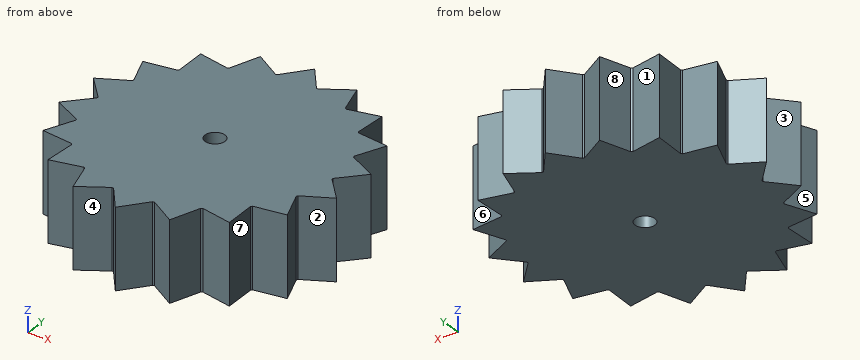
from build123d import *

# Parameters (mm, degrees)
F0_R     = 3.175
F1_DEPTH = 25.4


with BuildPart() as f1:
    # F0 (on Top) → F1 (new body)
    with BuildSketch(Plane.XY):
        with BuildLine():
            Line((0, 45.72), (-6.327913, 37.570833))
            ThreePointArc((-6.327913, 37.570833), (-6.615996, 37.521175), (-6.903689, 37.469309))
            Line((-6.903689, 37.469309), (-15.637161, 42.962747))
            Line((-15.637161, 42.962747), (-18.796275, 33.140761))
            ThreePointArc((-18.796275, 33.140761), (-19.05, 32.995568), (-19.302604, 32.848432))
            Line((-19.302604, 32.848432), (-29.38825, 35.023552))
            Line((-29.38825, 35.023552), (-28.997529, 24.713424))
            ThreePointArc((-28.997529, 24.713424), (-29.186293, 24.490208), (-29.37334, 24.26555))
            Line((-29.37334, 24.26555), (-39.594681, 22.86))
            Line((-39.594681, 22.86), (-35.701253, 13.305283))
            ThreePointArc((-35.701253, 13.305283), (-35.802289, 13.030967), (-35.901217, 12.755885))
            Line((-35.901217, 12.755885), (-45.02541, 7.939195))
            Line((-45.02541, 7.939195), (-38.098879, 0.292329))
            ThreePointArc((-38.098879, 0.292329), (-38.1, 0), (-38.098879, -0.292329))
            Line((-38.098879, -0.292329), (-45.02541, -7.939195))
            Line((-45.02541, -7.939195), (-35.901217, -12.755885))
            ThreePointArc((-35.901217, -12.755885), (-35.802289, -13.030967), (-35.701253, -13.305283))
            Line((-35.701253, -13.305283), (-39.594681, -22.86))
            Line((-39.594681, -22.86), (-29.37334, -24.26555))
            ThreePointArc((-29.37334, -24.26555), (-29.186293, -24.490208), (-28.997529, -24.713424))
            Line((-28.997529, -24.713424), (-29.38825, -35.023552))
            Line((-29.38825, -35.023552), (-19.302604, -32.848432))
            ThreePointArc((-19.302604, -32.848432), (-19.05, -32.995568), (-18.796275, -33.140761))
            Line((-18.796275, -33.140761), (-15.637161, -42.962747))
            Line((-15.637161, -42.962747), (-6.903689, -37.469309))
            ThreePointArc((-6.903689, -37.469309), (-6.615996, -37.521175), (-6.327913, -37.570833))
            Line((-6.327913, -37.570833), (0, -45.72))
            Line((0, -45.72), (6.327913, -37.570833))
            ThreePointArc((6.327913, -37.570833), (6.615996, -37.521175), (6.903689, -37.469309))
            Line((6.903689, -37.469309), (15.637161, -42.962747))
            Line((15.637161, -42.962747), (18.796275, -33.140761))
            ThreePointArc((18.796275, -33.140761), (19.05, -32.995568), (19.302604, -32.848432))
            Line((19.302604, -32.848432), (29.38825, -35.023552))
            Line((29.38825, -35.023552), (28.997529, -24.713424))
            ThreePointArc((28.997529, -24.713424), (29.186293, -24.490208), (29.37334, -24.26555))
            Line((29.37334, -24.26555), (39.594681, -22.86))
            Line((39.594681, -22.86), (35.701253, -13.305283))
            ThreePointArc((35.701253, -13.305283), (35.802289, -13.030967), (35.901217, -12.755885))
            Line((35.901217, -12.755885), (45.02541, -7.939195))
            Line((45.02541, -7.939195), (38.098879, -0.292329))
            ThreePointArc((38.098879, -0.292329), (38.1, 0), (38.098879, 0.292329))
            Line((38.098879, 0.292329), (45.02541, 7.939195))
            Line((45.02541, 7.939195), (35.901217, 12.755885))
            ThreePointArc((35.901217, 12.755885), (35.802289, 13.030967), (35.701253, 13.305283))
            Line((35.701253, 13.305283), (39.594681, 22.86))
            Line((39.594681, 22.86), (29.37334, 24.26555))
            ThreePointArc((29.37334, 24.26555), (29.186293, 24.490208), (28.997529, 24.713424))
            Line((28.997529, 24.713424), (29.38825, 35.023552))
            Line((29.38825, 35.023552), (19.302604, 32.848432))
            ThreePointArc((19.302604, 32.848432), (19.05, 32.995568), (18.796275, 33.140761))
            Line((18.796275, 33.140761), (15.637161, 42.962747))
            Line((15.637161, 42.962747), (6.903689, 37.469309))
            ThreePointArc((6.903689, 37.469309), (6.615996, 37.521175), (6.327913, 37.570833))
            Line((6.327913, 37.570833), (0, 45.72))
        make_face()
        Circle(F0_R, mode=Mode.SUBTRACT)
    extrude(amount=F1_DEPTH)


solid = f1.part
Build history of the part. All positions in model axes, mm. Face numbers are marked on the shaded views. A direction names the side the tool comes from. Round coordinates to 2 decimals unless told otherwise and drop trailing zeros. Write each loop counter-clockwise with the first axis right and the second up, starting at its lowest first coordinate (ties: lowest second). Pieces come first, ordered by that corner, then holes. Notation, with made-up numbers: M 83,86 L 98,86 A20 ccw 98,104 Z; hole C 76.5,57.25 d1. An arc over 180 degrees is marked long. Answer as a JSON object with one key per item and string values. Group by question number.
(1) Flat gauge pins, fed straight in: pin 1 (6 mm diameter, centred on x = 10, z = 17, fed in from -Y); pin 2 (6 mm diameter, centred on y = 12, z = 12, fed in from -X); pin 3 (3 mm diameter, centred on y = -31.5, z = 3, fed in from +X). Where does each tip first touch, or does it go through?
(2) Cut at B-B (y = -17.5). Give the cut face in (x, z).
(3) Drill centre lines: L1, parallel to Y at x = 0, z = 9.25 (3 decimals); L2, parallel to X at y = 41, z = 20.25; L3, parallel to Y at x = -40, z = 6. Where is each one in solid material? Low to high.
(4) Which spindle directions (+Z, -Z, +X, -X, +Y, -Y) get a long thin tool onto all of the face, cutting with end or side? Do the marked faces 4, 5, 6, 7 and 8. Say none if no direction does.
(5) Mould opens along X. For the marked faces 1, 2 and 3 say: pulls with the +X half, pulls with the -X half, needs draft (parallel to the pull), parting line crosses it, or undercut.
(6) Cut at A-A (x = 26). Give the cut face in (y, z).
Responses:
{
 "1": {"pin 1": "stops at y = -41.3", "pin 2": "stops at x = -43.02", "pin 3": "stops at x = 29.31"},
 "2": {"outline": "M -37.41,0 L 37.41,0 L 37.41,25.4 L -37.41,25.4 Z"},
 "3": {"L1": "y = -45.72 to -3.175, 3.175 to 45.72", "L2": "x = -16.27 to -12.52, -3.67 to 3.67, 12.52 to 16.27", "L3": "y = -10.59 to -2.39, 2.39 to 10.59"},
 "4": {"face 4": "+Z, -Z, -Y", "face 5": "+Z, -Z, -X", "face 6": "+Z, -Z, +X, +Y", "face 7": "+Z, -Z, +X", "face 8": "+Z, -Z, +Y"},
 "5": {"face 1": "undercut", "face 2": "pulls with the +X half", "face 3": "pulls with the -X half"},
 "6": {"outline": "M -34.29,0 L 34.29,0 L 34.29,25.4 L -34.29,25.4 Z"}
}
